from build123d import *

# Parameters (mm, degrees)
FASE1_SIZE                      = 2
FASE1_SIZE2                     = 3.464101615
SKIZZE2_W                       = 70
SKIZZE2_H                       = 45
SKIZZE2_R                       = 4.5
AUFSATZ_LINEAR_AUSTRAGEN1_DEPTH = 8


with BuildPart() as part:
    # Skizze1 → Rotation1 (revolve)
    with BuildSketch(Plane.XY):
        with BuildLine():
            Line((79.052558883, 0), (79.052558883, 4))
            Line((79.052558883, 4), (21.732050808, 4))
            ThreePointArc((21.732050808, 4), (19.143860357, 4.340741737), (16.732050808, 5.339745962))
            Line((16.732050808, 5.339745962), (0, 15))
            Line((0, 15), (0, 0))
            Line((0, 0), (79.052558883, 0))
        make_face()
    revolve(axis=Axis((0, 0, 0), (1, 0, 0)))

    # Fase1
    fase1_edges = [part.edges().sort_by_distance(p)[0] for p in [
        (79.052558883, -4, 0),
    ]]
    fase1_side = [part.faces().sort_by_distance(p)[0] for p in [
        (79.052558883, 0, 0),
    ]]
    chamfer(fase1_edges, length=FASE1_SIZE, length2=FASE1_SIZE2, reference=fase1_side[0])

    # Skizze2 → Aufsatz-Linear austragen1 (add)
    with BuildSketch(Plane.ZY):
        Rectangle(SKIZZE2_W, SKIZZE2_H)
        with Locations((-25, 0)):
            Circle(SKIZZE2_R, mode=Mode.SUBTRACT)
        with Locations((25, 0)):
            Circle(SKIZZE2_R, mode=Mode.SUBTRACT)
    extrude(amount=AUFSATZ_LINEAR_AUSTRAGEN1_DEPTH)


solid = part.part
Read the model definition and answer for the solid it produces. Units are mm, in the model's axes. A direction names the side the tool comes from. Round coordinates to 2 decimals unless told otherwise and drop trailing zeros. Loops run counter-clockwise (first coordinate to the right, second up) from the corner with the lowest first, then second, coordinate; pieces in that order, holes last.
Q1. Section B-B on y = 0 is taken. Write down the section's boundary in (x, z).
Q2. Consider probe 1 along Y at (x, z) = (-3, 25); probe 2 along X at (y, z) = (-12.5, -13); probe 3 along Y at (x, z) = (6, -9.5). Determine where each line is inside the solid, lowest interval first.
Q3. Section C-C on z = 0 is taken. Write down the section's boundary in (x, y), and give its area (3 significant figures).
Q4. Section A-A on z = 25 is taken. Write down the section's boundary in (x, y), and give its area (3 significant figures).
Q5. Each of these flat-tipped pins is pushed along its axis until it touches: pin 1 (3 mm diameter, centred on x = 29.5, z = 0.5, fed in from -Y); pin 2 (8 mm diameter, centred on y = 0, z = 25, fed in from -X); pin 3 (2 mm diameter, centred on x = 24, y = 4, fed in from +Z); pin 4 (3 mm diameter, centred on y = -12, z = -16, fed in from +X). Where does it stop, or does it pass through?
Q6. Determine the mould class of faces 1 (the face through (78.45, -1.86, -1.43)), 2 (the face through (79.053, 0, 0)), 3 (the face through (-3.944, 0.198, -29.496)) for opening direction Z: released by +Z, released by -Z, zero draft, split by the parting line, or undercut.
Q7. Section D-D on x = 71 is taken. Write down the section's boundary in (y, z), and give its area (3 significant figures).
Q8. Which of the six approach directions +Z, -Z, +X, -X, +Y, -Y give full straight-line access (tool end or side, diameter ignored) to faces 4 (the face through (48.283, -0.867, -3.905)), 5 (the face through (-4, 0, -35))?
Output:
1. outline: (-8, -35) - (0, -35) - (0, -29.5) - (-8, -29.5) - close; (-8, -20.5) - (0, -20.5) - (0, -15) - (16.73, -5.34) arc R10 cw to (21.73, -4) - (75.59, -4) - (79.05, -2) - (79.05, 2) - (75.59, 4) - (21.73, 4) arc R10 cw to (16.73, 5.34) - (0, 15) - (0, 20.5) - (-8, 20.5) - close; (-8, 29.5) - (0, 29.5) - (0, 35) - (-8, 35) - close
2. probe 1: y = -22.5 to -4.5, 4.5 to 22.5
2. probe 2: x = -8 to 0
2. probe 3: y = -6.54 to 6.54
3. outline: (-8, -22.5) - (0, -22.5) - (0, -15) - (16.73, -5.34) arc R10 cw to (21.73, -4) - (75.59, -4) - (79.05, -2) - (79.05, 2) - (75.59, 4) - (21.73, 4) arc R10 cw to (16.73, 5.34) - (0, 15) - (0, 22.5) - (-8, 22.5) - close
3. area: 1,200 mm2
4. outline: (-8, -22.5) - (0, -22.5) - (0, -4.5) - (-8, -4.5) - close; (-8, 4.5) - (0, 4.5) - (0, 22.5) - (-8, 22.5) - close
4. area: 288 mm2
5. pin 1: stops at y = -4
5. pin 2: passes through
5. pin 3: stops at z = 2.65
5. pin 4: stops at x = 0
6. face 1: split by the parting line
6. face 2: zero draft
6. face 3: undercut
7. outline: circle Ø8 at (0, 0)
7. area: 50.3 mm2
8. face 4: +X
8. face 5: -Z, +X, -X, +Y, -Y
